from build123d import *

# Parameters (mm, degrees)
F0_W     = 50.8
F0_H     = 50.8
F1_DEPTH = 6.35
F3_DEPTH = 6.35
F4_R     = 12.7
F5_DEPTH = 6.35
F6_R     = 1.5875


with BuildPart() as f1:
    # F0 (on Top) → F1 (new body)
    with BuildSketch(Plane.XY):
        Rectangle(F0_W, F0_H)
    extrude(amount=F1_DEPTH)

    # F2 (on face) → F3 (join)
    with BuildSketch(Plane.XY.offset(6.35)):
        Polygon((0, -25.4), (25.4, 0), (0, 25.4), (-25.4, 0), align=None)
    extrude(amount=F3_DEPTH)

    # F4 (on face) → F5 (join)
    with BuildSketch(Plane.XY.offset(12.7)):
        Circle(F4_R)
    extrude(amount=F5_DEPTH)

    # F6
    f6_edges = [f1.edges().sort_by_distance(p)[0] for p in [
        (-25.4, 0, 9.525),
        (25.4, 0, 9.525),
        (0, 25.4, 9.525),
        (0, -25.4, 9.525),
        (-25.4, 25.4, 3.175),
        (-25.4, -25.4, 3.175),
        (25.4, -25.4, 3.175),
        (25.4, 25.4, 3.175),
    ]]
    fillet(f6_edges, radius=F6_R)


solid = f1.part
Design review of the part built by this model. Coordinates are the model's own, in mm. A direction names the side the tool comes from. Coordinates: 2 decimals unless noted, no trailing zeros. Loops run counter-clockwise (first coordinate to the right, second up) from the corner with the lowest first, then second, coordinate; pieces in that order, holes last.
Item 1: Add section B-B (z = 12). Write out the cut boundary in (x, y) (1 decimal).
Completed:
outline: (-24.3, -1.1) - (-1.1, -24.3) arc R1.6 ccw to (1.1, -24.3) - (24.3, -1.1) arc R1.6 ccw to (24.3, 1.1) - (1.1, 24.3) arc R1.6 ccw to (-1.1, 24.3) - (-24.3, 1.1) arc R1.6 ccw to start
Item 2: Add section C-C (x = 0). Write out the cut boundary in (y, z), and give its area (3 significant figures).
Completed:
outline: (-25.4, 0) - (25.4, 0) - (25.4, 6.35) - (24.74, 6.35) - (24.74, 12.7) - (12.7, 12.7) - (12.7, 19.05) - (-12.7, 19.05) - (-12.7, 12.7) - (-24.74, 12.7) - (-24.74, 6.35) - (-25.4, 6.35) - close
area: 798 mm2
Item 3: Wall thickness on L1, parallel to Z at x = -4, y = 15.5; L2, parallel to Z at x = -18, y = -18; L3, parallel to Y at x = 0.5, z = 14: over which ranges is each line inside the solid? List them lowest first.
Completed:
L1: z = 0 to 12.7
L2: z = 0 to 6.35
L3: y = -12.69 to 12.69
Item 4: For faces 1 (the cylindrical face through (24.742, -0.017, 9.569)), 2 (the cylindrical face through (-24.742, -0.017, 9.569)), 3 (the flat face through (-12.5, 12.9, 9.5)), list the 3-axis set-ups (+Z, -Z, +X, -X, +Y, -Y) from which the entire face can be reached by the end or side of a thin tool; tool diameter is ignored.
Completed:
face 1: +Z, +X
face 2: +Z, -X
face 3: +Z, -X, +Y
Item 5: Clearance check with flat-ended pins moving along their axes: pin 1 (4 mm diameter, centred on x = 12.5, y = 17, fed in from +Z); pin 2 (2 mm diameter, centred on x = 19.5, y = -7, fed in from +Z); pin 3 (15 mm diameter, centred on x = -8, y = -10.5, fed in from +Z); pin 4 (2 mm diameter, centred on x = -8.5, z = 11, fed in from -Y). State where each tip first meets the part, or that it passes through.
Completed:
pin 1: stops at z = 6.35
pin 2: stops at z = 12.7
pin 3: stops at z = 19.05
pin 4: stops at y = -17.9
Item 6: Add section A-A (y = 20). Write out the cut boundary in (x, z), and give its area (3 significant figures).
Completed:
outline: (-25.4, 0) - (25.4, 0) - (25.4, 6.35) - (5.4, 6.35) - (5.4, 12.7) - (-5.4, 12.7) - (-5.4, 6.35) - (-25.4, 6.35) - close
area: 391 mm2
